from build123d import *

# Parameters (mm, degrees)
F0_R          = 62.5
F0_R_2        = 100
F1_DEPTH      = 10
F2_R          = 62.5
F2_R_2        = 45
F2_R_3        = 100
F2_R_4        = 77.5
F3_DEPTH      = 15
F3_DEPTH_BACK = 10
F5_DEPTH      = 7
F6_R          = 5


with BuildPart() as f1:
    # F0 (on Front) → F1 (new body)
    with BuildSketch(Plane.XZ):
        with BuildLine():
            Line((-335.641221, -67.007242), (-12.905344, -106.218888))
            ThreePointArc((-12.905344, -106.218888), (106.999999, 0.015565), (-12.936245, 106.215129))
            Line((-12.936245, 106.215129), (-339.19516, 66.479119))
            ThreePointArc((-339.19516, 66.479119), (-394.976089, -1.796482), (-335.641221, -67.007242))
        make_face()
        with Locations((-327.5, 0)):
            Circle(F0_R, mode=Mode.SUBTRACT)
        Circle(F0_R_2, mode=Mode.SUBTRACT)
    extrude(amount=F1_DEPTH)

    # F2 (on face) → F3 (join, two sides)
    with BuildSketch(Plane.XZ.offset(10)) as f3_sk:
        with Locations((-327.5, 0)):
            Circle(F2_R)
        with Locations((-327.5, 0)):
            Circle(F2_R_2, mode=Mode.SUBTRACT)
        Circle(F2_R_3)
        Circle(F2_R_4, mode=Mode.SUBTRACT)
    extrude(amount=F3_DEPTH)
    extrude(f3_sk.sketch, amount=-F3_DEPTH_BACK)

    # F4 (on face) → F5 (cut)
    with BuildSketch(Plane.XZ.offset(10)):
        with BuildLine():
            ThreePointArc((-66.577581, -82.482881), (-105.999999, -0.015419), (-66.601576, 82.463508))
            ThreePointArc((-66.601576, 82.463508), (-64.845792, 89.469376), (-71.096873, 93.087242))
            Line((-71.096873, 93.087242), (-285.484696, 66.976334))
            ThreePointArc((-285.484696, 66.976334), (-290.580254, 62.475162), (-288.201504, 56.105955))
            ThreePointArc((-288.201504, 56.105955), (-259.000022, -0.055148), (-288.291894, -56.169159))
            ThreePointArc((-288.291894, -56.169159), (-290.67952, -62.540062), (-285.581272, -67.045285))
            Line((-285.581272, -67.045285), (-71.069788, -93.107923))
            ThreePointArc((-71.069788, -93.107923), (-64.81976, -89.488238), (-66.577581, -82.482881))
        make_face()
    extrude(amount=-F5_DEPTH, mode=Mode.SUBTRACT)

    # F6
    f6_edges = [f1.edges().sort_by_distance(p)[0] for p in [
        (-105.999999, -3, -0.015419),
    ]]
    fillet(f6_edges, radius=F6_R)


solid = f1.part
Geometry: final body of the model. Coordinates: model frame, mm. A direction names the side the tool comes from. Round coordinates to 2 decimals unless told otherwise and drop trailing zeros. Order: outer loops, then holes, each group sorted by start corner. A loop starts at its lowest first (then second) coordinate and runs counter-clockwise, first axis right, second up.
Q1. Pin query (flat end, axial travel): pin 1 (12 mm diameter, centred on x = -174, y = -19, fed in from +Z); pin 2 (8 mm diameter, centred on y = -7.5, z = -75, fed in from +X); pin 3 (8 mm diameter, centred on x = -192, y = -13.5, fed in from +Z); pin 4 (6 mm diameter, centred on x = -248.5, y = -11.5, fed in from +Z). Return the tip coordinate at first contact, or that it passes through.
Result sheet:
pin 1: passes through
pin 2: stops at x = 80.05
pin 3: stops at z = 84.64
pin 4: stops at z = 77.84
Q2. Mould query, pull axis X, two halves, no side actions, for faces 1 (the face through (-176.79, -9.014, 80.215)), 2 (the face through (-173.782, -4.93, 86.625)), 3 (the face through (-284.58, -12.32, 13.52)), 4 (the face through (-342, -25, 43)). Classes: released by +X, released by -X, zero draft, split by the parting line, or undercut.
Result sheet:
face 1: undercut
face 2: released by -X
face 3: undercut
face 4: zero draft
Q3. Section C-C, the plane y = -17. Output: boundary loops of the cut face in (x, z).
Result sheet:
outline: circle Ø125 at (-327.5, 0); circle Ø200 at (0, 0); hole circle Ø90 at (-327.5, 0); hole circle Ø155 at (0, 0)
Q4. Section D-D, the plane x = -327.5. Output: boundary loops of the cut face in (y, z), and give its area (3 significant figures).
Result sheet:
outline: (-25, -62.5) - (-10, -62.5) - (-10, -68) - (0, -68) - (0, -45) - (-25, -45) - close; (-25, 45) - (0, 45) - (0, 67.9) - (-10, 67.9) - (-10, 62.5) - (-25, 62.5) - close
area: 984 mm2
Q5. Section B-B, the plane z = 0. Give the number of separate pieces and of enclosed holes in the cut face, and give its area (3 significant figures).
Result sheet:
separate pieces: 3
enclosed holes: 0
area: 2,710 mm2
Q6. Access query for faces 5 (the face through (-395, -5, 0)), 6 (the face through (95.38, -17.4, 30.04)). Directions: +Z, -Z, +X, -X, +Y, -Y. A direction counts if a zero-diameter tool reaches every point of the face in a straight line with its end or side. Return the directions, or none.
Result sheet:
face 5: -X, +Y, -Y
face 6: -Y
Q7. Section A-A, the plane x = 0. Output: boundary loops of the cut face in (y, z).
Result sheet:
outline: (-25, -100) - (-10, -100) - (-10, -107) - (0, -107) - (0, -77.5) - (-25, -77.5) - close; (-25, 77.5) - (0, 77.5) - (0, 107) - (-10, 107) - (-10, 100) - (-25, 100) - close
Q8. Material intervals for probe 1 along Z at (x, y) = (-279, -9.75); probe 2 along Z at (x, y) = (-327.5, -18.75); probe 3 along X at (y, z) = (-17.75, -53), sorted ascending.
Result sheet:
probe 1: z = -73.89 to -67.84, -48.37 to 48.37, 67.77 to 73.81
probe 2: z = -62.5 to -45, 45 to 62.5
probe 3: x = -360.62 to -294.38, -84.8 to -56.54, 56.54 to 84.8
